Geometry: final body of the model. Coordinates: model frame, mm. Face numbers are marked on the shaded views. A direction names the side the tool comes from. Round coordinates to 2 decimals unless told otherwise and drop trailing zeros. Loops run counter-clockwise (first coordinate to the right, second up) from the corner with the lowest first, then second, coordinate; pieces in that order, holes last. Notation, with made-up numbers: (26, 72.5) -> (33, 72.5) arc R12 ccw to (33, 78.5) -> close; hole circle Ø1 at (60.25, 72.5). An arc over 180 degrees is marked (long way). Answer in a Markdown table with one row per item.
```python
from build123d import *

# Parameters (mm, degrees)
SKETCH1_R           = 10
BOSS_EXTRUDE1_DEPTH = 10
SKETCH3_R           = 5
BOSS_EXTRUDE2_DEPTH = 8
SKETCH4_R           = 3
CUT_EXTRUDE1_DEPTH  = 27
SKETCH5_R           = 1.5
CUT_EXTRUDE2_DEPTH  = 27


with BuildPart() as part:
    # Sketch1 → Boss-Extrude1 (new body)
    with BuildSketch(Plane.XY):
        Circle(SKETCH1_R)
    extrude(amount=BOSS_EXTRUDE1_DEPTH)

    # Sketch3 → Boss-Extrude2 (add)
    with BuildSketch(Plane(origin=(0, 0, 0), x_dir=(-1, 0, 0), z_dir=(0, 0, -1))):
        with Locations(Location((0, 0, 0), (0, 0, 180))):
            Circle(SKETCH3_R)
    extrude(amount=BOSS_EXTRUDE2_DEPTH)

    # Sketch4 → Cut-Extrude1 (cut)
    with BuildSketch(Plane(origin=(0, 0, -8), x_dir=(-1, 0, 0), z_dir=(0, 0, -1))):
        Circle(SKETCH4_R)
    extrude(amount=-CUT_EXTRUDE1_DEPTH, mode=Mode.SUBTRACT)

    # Sketch5 → Cut-Extrude2 (cut)
    with BuildSketch(Plane(origin=(0, 0, 0), x_dir=(1, 0, 0), z_dir=(0, 1, 0))):
        with Locations(Location((0, 5, 0), (0, 0, 270))):
            Circle(SKETCH5_R)
    extrude(amount=-CUT_EXTRUDE2_DEPTH, mode=Mode.SUBTRACT)


solid = part.part
```
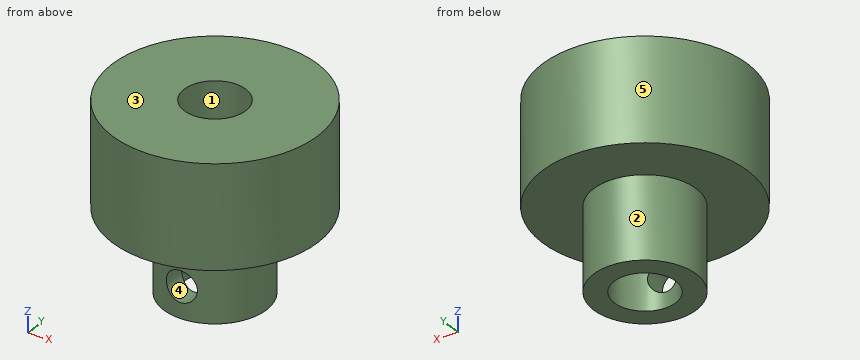
Item 1: Cut plane B-B (x = 0). Output: boundary loops of the cut face in (y, z).
Answer:
| item | result |
|---|---|
| outline | (-10, 0) -> (-5, 0) -> (-5, -3.5) -> (-3, -3.5) -> (-3, 10) -> (-10, 10) -> close; (-5, -8) -> (-3, -8) -> (-3, -6.5) -> (-5, -6.5) -> close; (3, -8) -> (5, -8) -> (5, 0) -> (10, 0) -> (10, 10) -> (3, 10) -> close |
Item 2: Cut plane D-D (z = 2.25). Output: boundary loops of the cut face in (x, y), then the cut area to 3 significant figures.
Answer:
| item | result |
|---|---|
| outline | circle Ø20 at (0, 0); hole circle Ø6 at (0, 0) |
| area | 286 mm² |
Item 3: Line query: probe 1 along Y at (x, z) = (0, -2.25); probe 2 along Z at (x, y) = (0, -3.1); probe 3 along Z at (x, y) = (-0.5, -5.75). Output: solid intervals per line, ascending. Write a range as [from, to].
Answer:
| item | result |
|---|---|
| probe 1 | y = [-5, -3], [3, 5] |
| probe 2 | z = [-8, -6.5], [-3.5, 10] |
| probe 3 | z = [0, 10] |
Item 4: Pin query (flat end, axial travel): pin 1 Ø8 at (x, y) = (5, 7) entering from -Z; pin 2 Ø3.5 at (x, z) = (0, -5) entering from -Y; pin 3 Ø1.5 at (y, z) = (5, -3.5) entering from +X; pin 4 Ø1.5 at (y, z) = (-7, -0.5) entering from +X. Return the tip coordinate at first contact, or that it passes through.
Answer:
| item | result |
|---|---|
| pin 1 | stops at z = -8 |
| pin 2 | stops at y = -5 |
| pin 3 | stops at x = 2.63 |
| pin 4 | stops at x = 7.65 |
Item 5: Reachability of the marked faces 1 and 2 from +Z, -Z, +X, -X, +Y, -Y: full face, straight path, thin tool, end or side. Return the list, or none.
Answer:
| item | result |
|---|---|
| face 1 | +Z, -Z |
| face 2 | -Z |
Item 6: Draft query along Z for the marked faces 3, 4 and 5. Return one class per face: pulls with the +Z half, pulls with the -Z half, needs draft (parallel to the pull), parting line crosses it, or undercut.
Answer:
| item | result |
|---|---|
| face 3 | pulls with the +Z half |
| face 4 | undercut |
| face 5 | needs draft |
Item 7: Cut plane A-A (y = 0). Output: boundary loops of the cut face in (x, z).
Answer:
| item | result |
|---|---|
| outline | (-10, 0) -> (-5, 0) -> (-5, -8) -> (-3, -8) -> (-3, 10) -> (-10, 10) -> close; (3, -8) -> (5, -8) -> (5, 0) -> (10, 0) -> (10, 10) -> (3, 10) -> close |
Item 8: Cut plane C-C (y = -4). Output: boundary loops of the cut face in (x, z), then the cut area to 3 significant figures.
Answer:
| item | result |
|---|---|
| outline | (-9.17, 0) -> (-3, 0) -> (-3, -8) -> (3, -8) -> (3, 0) -> (9.17, 0) -> (9.17, 10) -> (-9.17, 10) -> close; hole circle Ø3 at (0, -5) |
| area | 224 mm² |
